```python
from build123d import *

# Parameters (mm, degrees)
F0_R     = 19.05
F1_DEPTH = 31.75
F3_R     = 5.5626
F4_DEPTH = 4.7752
F5_DEPTH = 57.151


with BuildPart() as f1:
    # F0 (on Front) → F1 (new body, symmetric)
    with BuildSketch(Plane.XZ):
        with BuildLine():
            Line((102.1447438789, 28.575), (0, 28.575))
            ThreePointArc((0, 28.575), (-20.2055762724, -20.2055762724), (28.575, 0))
            ThreePointArc((28.575, 0), (29.7781261877, 8.674261314), (37.5552561211, 12.7))
            Line((37.5552561211, 12.7), (102.1447438789, 12.7))
            Line((102.1447438789, 12.7), (102.1447438789, 28.575))
        make_face()
        Circle(F0_R, mode=Mode.SUBTRACT)
    extrude(amount=F1_DEPTH, both=True)

    # F3 (on face) → F4 (join)
    with BuildSketch(Plane.XY.offset(28.575)):
        with BuildLine():
            ThreePointArc((44.2432574162, 31.75), (38.9330700337, 26.4354220023), (37.5552561211, 19.05))
            Line((37.5552561211, 19.05), (37.5552561211, -19.05))
            ThreePointArc((37.5552561211, -19.05), (38.9330700337, -26.4354220023), (44.2432574161, -31.75))
            Line((44.2432574161, -31.75), (56.097272461, -31.75))
            Line((56.097272461, -31.75), (95.3253515684, -11.2564849399))
            ThreePointArc((95.3253515684, -11.2564849399), (100.3069194614, -6.5805122609), (102.1447438789, -7.87e-08))
            ThreePointArc((102.1447438789, -7.87e-08), (100.3069195022, 6.5805121935), (95.3253515684, 11.2564849399))
            Line((95.3253515684, 11.2564849399), (56.097272461, 31.75))
            Line((56.097272461, 31.75), (44.2432574162, 31.75))
        make_face()
        with Locations((50.170148764, -20.5178159314)):
            Circle(F3_R, mode=Mode.SUBTRACT)
        with Locations((50.170148764, 20.5178159314)):
            Circle(F3_R, mode=Mode.SUBTRACT)
        with Locations((89.4447438789, 0)):
            Circle(F3_R, mode=Mode.SUBTRACT)
    extrude(amount=F4_DEPTH)

    # F5 (cut, through all): faces of the model
    f5_faces = [f1.faces().sort_by_distance(p)[0] for p in [
        (89.4447438789, 0, 28.575),
        (50.170148764, -20.5178159314, 28.575),
        (50.170148764, 20.5178159314, 28.575),
    ]]
    extrude(f5_faces, amount=-F5_DEPTH, mode=Mode.SUBTRACT)


solid = f1.part
```
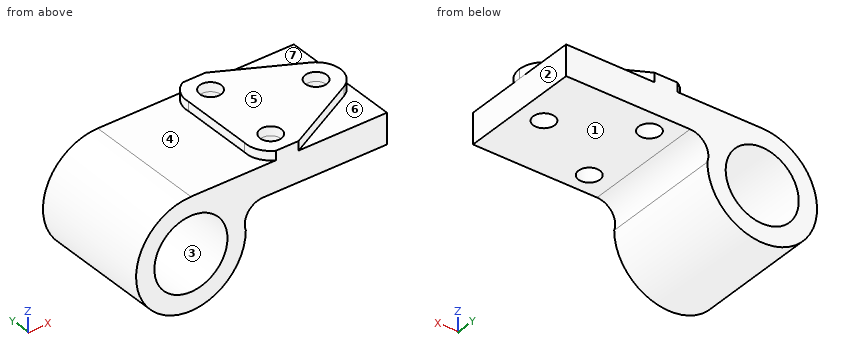
Design review of the part built by this model. Coordinates are the model's own, in mm. Face numbers are marked on the shaded views. A direction names the side the tool comes from. Coordinates: 2 decimals unless noted, no trailing zeros. Write each loop counter-clockwise with the first axis right and the second up, starting at its lowest first coordinate (ties: lowest second). Pieces come first, ordered by that corner, then holes.
1) Add section D-D (z = -11.5). Write out the cut boundary in (x, y), plus the area to 3 significant figures.
2) Add section A-A (y = 23). Write out the cut boundary in (x, z) (3 decimals).
3) Add section C-C (x = 14.5). Write out the cut boundary in (y, z) (3 decimals), plus the area to 3 significant figures.
4) Add section B-B (z = 17). Write out the cut boundary in (x, y), plus the area to 3 significant figures.
5) Machinability: for the marked faces 5, 6 and 7, which of the approach directions +Z, -Z, +X, -X, +Y, -Y give a long, thin tool a straight path to every point of the face, cutting with its end or side? Answer none if there is none.
6) To check wall thickness, follow L1, parallel to Z at x = 0, y = -13 (3 decimals); L2, parallel to X at y = 16.5, z = 14.5; L3, parallel to Z at x = 65, y = -6.5. State the ranges of each line that lie inside material, in increasing order.
7) Mouldability with a two-part tool opening along Z and no side actions: class the marked faces 1, 2, 3 and 4 as +Z half, -Z half, draft (parallel to the pull), parting line (faces both ways), or undercut.
8) Insertion check: pin 1 (10 mm diameter, centred on x = 13, y = 19.5, fed in from +Z) (3 decimals); pin 2 (3 mm diameter, centred on y = -8.5, z = 15.5, fed in from -X); pin 3 (14.5 mm diameter, centred on x = 50.17, y = 20.52, fed in from +Z); pin 4 (4 mm diameter, centred on x = 89, y = -9.5, fed in from -Z). Each pin has a flat end and moves straight along its axis. Give the tip position at first contact, or say it passes through.
Check result:
1. outline: (-26.16, -31.75) - (-15.19, -31.75) - (-15.19, 31.75) - (-26.16, 31.75) - close; (15.19, -31.75) - (26.16, -31.75) - (26.16, 31.75) - (15.19, 31.75) - close
1. area: 1,390 mm2
2. outline: (0, 28.575) arc R28.575 ccw (long way) to (28.575, 0) arc R9.525 cw to (37.555, 12.7) - (45.192, 12.7) - (45.192, 33.35) - (37.715, 33.35) - (37.715, 28.575) - close; (55.148, 12.7) - (102.145, 12.7) - (102.145, 28.575) - (72.846, 28.575) - (72.846, 33.35) - (55.148, 33.35) - close; hole circle Ø38.1 at (0, 0)
3. outline: (-31.75, -24.623) - (31.75, -24.623) - (31.75, -12.355) - (-31.75, -12.355) - close; (-31.75, 12.355) - (31.75, 12.355) - (31.75, 28.575) - (-31.75, 28.575) - close
3. area: 1,810 mm2
4. outline: (-22.97, -31.75) - (-8.6, -31.75) - (-8.6, 31.75) - (-22.97, 31.75) - close; (8.6, -31.75) - (102.14, -31.75) - (102.14, 31.75) - (8.6, 31.75) - close; hole circle Ø11.13 at (50.17, -20.52); hole circle Ø11.13 at (50.17, 20.52); hole circle Ø11.13 at (89.44, 0)
4. area: 6,560 mm2
5. face 5: +Z, +X, -X, +Y, -Y
5. face 6: +Z, +X, -Y
5. face 7: +Z, +X, +Y
6. L1: z = -28.575 to -19.05, 19.05 to 28.575
6. L2: x = -24.62 to -12.36, 12.36 to 46.32, 54.02 to 102.14
6. L3: z = 12.7 to 33.35
7. face 1: -Z half
7. face 2: draft
7. face 3: undercut
7. face 4: +Z half
8. pin 1: stops at z = 28.575
8. pin 2: stops at x = -24.91
8. pin 3: stops at z = 33.35
8. pin 4: stops at z = 12.7
